Work out the finished part from the listing and answer in its coordinate system (mm). Face numbers are marked on the shaded views. A direction names the side the tool comes from. Give positions to 0.01 mm unless a question says otherwise; leave off trailing zeros. Loops run counter-clockwise (first coordinate to the right, second up) from the corner with the lowest first, then second, coordinate; pieces in that order, holes last.
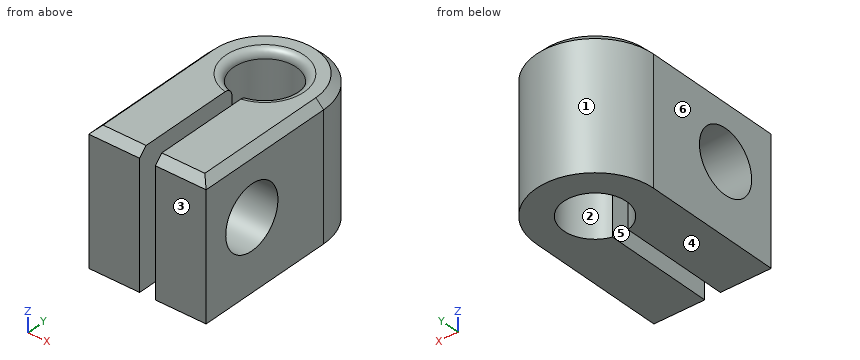
from build123d import *

# Parameters (mm, degrees)
BOX001_W                = 2
BOX001_H                = 17
BOX001_DEPTH            = 17
CYLINDER002_R           = 4
CYLINDER002_DEPTH       = 15
CYLINDER002_PITCH_ANGLE = 90
CYLINDER001_R           = 4
CYLINDER001_DEPTH       = 17
BOX_W                   = 15
BOX_H                   = 18
BOX_DEPTH               = 17
CYLINDER_R              = 7.5
CYLINDER_DEPTH          = 17
CHAMFER_SIZE            = 1
FILLET_R                = 1


with BuildPart() as box001:
    # Box001 → Box001 (new body)
    with BuildSketch(Plane(origin=(6.5, 0, 0), x_dir=(1, 0, 0), z_dir=(0, 0, 1))):
        with Locations((1, 8.5)):
            Rectangle(BOX001_W, BOX001_H)
    extrude(amount=BOX001_DEPTH)


with BuildPart() as cylinder002:
    # Cylinder002 → Cylinder002 (new body)
    with BuildSketch(Plane.XY):
        Circle(CYLINDER002_R)
    extrude(amount=CYLINDER002_DEPTH)


with BuildPart() as cylinder002_1:
    # Cylinder002 pitch: moved
    add(cylinder002.part.rotate(Axis((0, 0, 0), (0, 1, 0)), CYLINDER002_PITCH_ANGLE))


with BuildPart() as cylinder002_2:
    # Cylinder002 placement: moved
    add(cylinder002_1.part.moved(Location((0, 7, 9))))


with BuildPart() as cylinder001:
    # Cylinder001 → Cylinder001 (new body)
    with BuildSketch(Plane(origin=(7.5, 18, 0), x_dir=(1, 0, 0), z_dir=(0, 0, 1))):
        Circle(CYLINDER001_R)
    extrude(amount=CYLINDER001_DEPTH)


with BuildPart() as box:
    # Box → Box (new body)
    with BuildSketch(Plane.XY):
        with Locations((7.5, 9)):
            Rectangle(BOX_W, BOX_H)
    extrude(amount=BOX_DEPTH)


with BuildPart() as fillet_body:
    # Cylinder → Cylinder (new body)
    with BuildSketch(Plane(origin=(7.5, 18, 0), x_dir=(1, 0, 0), z_dir=(0, 0, 1))):
        Circle(CYLINDER_R)
    extrude(amount=CYLINDER_DEPTH)

    # Fusion: union Box
    add(box.part)

    # Cut: cut Cylinder001
    add(cylinder001.part, mode=Mode.SUBTRACT)

    # Cut001: cut Cylinder002
    add(cylinder002_2.part, mode=Mode.SUBTRACT)

    # Cut002: cut Box001
    add(box001.part, mode=Mode.SUBTRACT)

    # Chamfer
    chamfer_edges = [fillet_body.edges().sort_by_distance(p)[0] for p in [
        (3.25, 0, 17),
        (0, 9, 17),
        (7.5, 25.5, 17),
        (15, 9, 17),
        (11.75, 0, 17),
    ]]
    chamfer(chamfer_edges, length=CHAMFER_SIZE)

    # Fillet
    fillet_edges = [fillet_body.edges().sort_by_distance(p)[0] for p in [
        (4.337722, 15.55051, 17),
        (7.5, 22, 17),
        (10.662278, 15.55051, 17),
    ]]
    fillet(fillet_edges, radius=FILLET_R)


solid = fillet_body.part
Item 1: Find section B-B, the plane y = 12.75. Write down the section's boundary in (x, z), plus the area to 3 significant figures.
Item 2: For the marked faces 5 and 6, determine the directions among +Z, -Z, +X, -X, +Y, -Y from which every point of the face is accessible in a straight line to the end or side of a thin tool.
Item 3: Determine the mould class of the marked faces 1, 2, 3 and 4 for opening direction Y: released by +Y, released by -Y, zero draft, split by the parting line, or undercut.
Item 4: Consider line 1 (X direction, y = 13, z = 8.5); line 2 (Y direction, x = 4.5, z = 9); line 3 (X direction, y = 18, z = 12.5). Determine where each line is inside the solid, lowest interval first.
Item 5: Find section A-A, the plane z = 9. Write down the section's boundary in (x, y), plus the area to 3 significant figures.
Item 6: A flat-ended cylindrical pin translates along its axis: pin 1 Ø7 at (y, z) = (10, 6.5) entering from -X. Find the tip coordinate at first contact, or state that the pin passes through.
Item 7: Find section C-C, the plane y = 7. Write down the section's boundary in (x, z).
Item 8: Find section D-D, the plane x = 7.5. Write down the section's boundary in (y, z).
Ans:
1. outline: (0, 0) - (6.5, 0) - (6.5, 17) - (1, 17) - (0, 16) - close; (8.5, 0) - (15, 0) - (15, 16) - (14, 17) - (8.5, 17) - close
1. area: 220 mm2
2. face 5: +Z, -Z, -Y
2. face 6: +Z, -Z, -X, +Y, -Y
3. face 1: released by +Y
3. face 2: undercut
3. face 3: released by -Y
3. face 4: zero draft
4. line 1: x = 0 to 6.5, 8.5 to 15
4. line 2: y = 0 to 3, 11 to 15.35, 20.65 to 24.87
4. line 3: x = 0 to 3.5, 11.5 to 15
5. outline: (0, 0) - (6.5, 0) - (6.5, 3) - (0, 3) - close; (0, 11) - (6.5, 11) - (6.5, 14.13) arc R4 cw (long way) to (8.5, 14.13) - (8.5, 11) - (15, 11) - (15, 18) arc R7.5 ccw to (0, 18) - close; (8.5, 0) - (15, 0) - (15, 3) - (8.5, 3) - close
5. area: 176 mm2
6. pin 1: stops at x = 0
7. outline: (0, 0) - (6.5, 0) - (6.5, 5) - (0, 5) - close; (0, 13) - (6.5, 13) - (6.5, 17) - (1, 17) - (0, 16) - close; (8.5, 0) - (15, 0) - (15, 5) - (8.5, 5) - close; (8.5, 13) - (15, 13) - (15, 16) - (14, 17) - (8.5, 17) - close
8. outline: (22, 0) - (25.5, 0) - (25.5, 16) - (24.5, 17) - (23, 17) arc R1 ccw to (22, 16) - close
